Can you work these out from the model? Positions are in its coordinate system, mm. Face numbers are marked on the shaded views. A direction names the side the tool comes from. Give positions to 0.01 mm unless a question says otherwise; leave off trailing zeros. Loops run counter-clockwise (first coordinate to the right, second up) from the corner with the lowest first, then second, coordinate; pieces in that order, holes last.
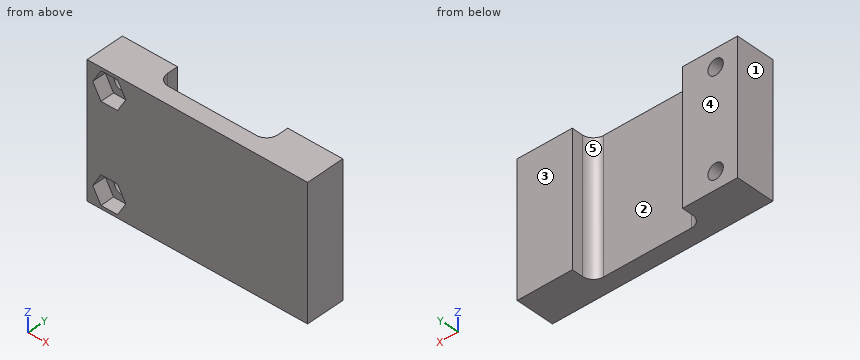
from build123d import *

# Parameters (mm, degrees)
SKETCH1_W           = 40
SKETCH1_H           = 24
SKETCH1_R           = 1.4
BOSS_EXTRUDE1_DEPTH = 7
SKETCH2_W           = 20
SKETCH2_H           = 24
CUT_EXTRUDE1_DEPTH  = 4
FILLET1_R           = 2
CUT_EXTRUDE2_DEPTH  = 2.5


with BuildPart() as part:
    # Sketch1 → Boss-Extrude1 (new body)
    with BuildSketch(Plane(origin=(0, 0, 0), x_dir=(1, 0, 0), z_dir=(0, 1, 0))):
        Rectangle(SKETCH1_W, SKETCH1_H)
        with Locations(Location((-16, 8.825, 0), (0, 0, 270))):
            Circle(SKETCH1_R, mode=Mode.SUBTRACT)
        with Locations(Location((-16, -8.825, 0), (0, 0, 270))):
            Circle(SKETCH1_R, mode=Mode.SUBTRACT)
    extrude(amount=BOSS_EXTRUDE1_DEPTH)

    # Sketch2 → Cut-Extrude1 (cut)
    with BuildSketch(Plane(origin=(0, 7, 0), x_dir=(1, 0, 0), z_dir=(0, 1, 0))):
        Rectangle(SKETCH2_W, SKETCH2_H)
    extrude(amount=-CUT_EXTRUDE1_DEPTH, mode=Mode.SUBTRACT)

    # Fillet1
    fillet1_edges = [part.edges().sort_by_distance(p)[0] for p in [
        (-10, 3, 0),
        (10, 3, 0),
    ]]
    fillet(fillet1_edges, radius=FILLET1_R)

    # Sketch3 → Cut-Extrude2 (cut)
    with BuildSketch(Plane.XZ):
        Polygon((-14.4988893, 6.225), (-12.9977786, 8.825), (-14.4988893, 11.425), (-17.5011107, 11.425), (-19.0022214, 8.825), (-17.5011107, 6.225), align=None)
        Polygon((-14.4988893, -11.425), (-12.9977786, -8.825), (-14.4988893, -6.225), (-17.5011107, -6.225), (-19.0022214, -8.825), (-17.5011107, -11.425), align=None)
    extrude(amount=-CUT_EXTRUDE2_DEPTH, mode=Mode.SUBTRACT)


solid = part.part
(1) Suppose I cut it at D-D on z = 9.75. List the corners of the cut face in (x, y) for me, plus the area to 3 significant figures.
Returned:
outline: (-20, 0) - (-18.47, 0) - (-18.47, 2.5) - (-17.05, 2.5) - (-17.05, 7) - (-20, 7) - close; (-14.95, 2.5) - (-13.53, 2.5) - (-13.53, 0) - (20, 0) - (20, 7) - (10, 7) - (10, 5) arc R2 cw to (8, 3) - (-8, 3) arc R2 cw to (-10, 5) - (-10, 7) - (-14.95, 7) - close
area: 180 mm2
(2) Will these pins go through, and if not, where does the flat tip stop? P1, Ø5, axis at x = 2.5, z = 5.5, coming from the +Y side; P2, Ø1.5, axis at x = 8.5, z = 7, coming from the -Y side; P3, Ø4.5, axis at x = -16, z = -8.825, coming from the -Y side; P4, Ø2.5, axis at x = -16, z = 8.825, coming from the +Y side.
Returned:
P1: stops at y = 3
P2: stops at y = 0
P3: stops at y = 2.5
P4: passes through
(3) Thinking about a two-plate mould opening in X: for the marked faces 1, 2 and 3, which applies, pulls with the +X half, pulls with the -X half, needs draft (parallel to the pull), parting line crosses it, or undercut?
Returned:
face 1: pulls with the -X half
face 2: undercut
face 3: needs draft
(4) Suppose I cut it at A-A on y = 6.25. List the corners of the cut face in (x, z) for me (3 decimals).
Returned:
outline: (-20, -12) - (-10, -12) - (-10, 12) - (-20, 12) - close; (10, -12) - (20, -12) - (20, 12) - (10, 12) - close; hole circle Ø2.8 at (-16, -8.825); hole circle Ø2.8 at (-16, 8.825)
(5) Suppose I cut it at B-B on x = -16. List the corners of the cut face in (y, z) for me (3 decimals).
Returned:
outline: (0, -12) - (7, -12) - (7, -10.225) - (2.5, -10.225) - (2.5, -11.425) - (0, -11.425) - close; (0, -6.225) - (2.5, -6.225) - (2.5, -7.425) - (7, -7.425) - (7, 7.425) - (2.5, 7.425) - (2.5, 6.225) - (0, 6.225) - close; (0, 11.425) - (2.5, 11.425) - (2.5, 10.225) - (7, 10.225) - (7, 12) - (0, 12) - close
(6) Suppose I cut it at C-C on y = 1.25. List the corners of the cut face in (x, z) for me (3 decimals), plus the area to 3 significant figures.
Returned:
outline: (-20, -12) - (20, -12) - (20, 12) - (-20, 12) - close; hole (-19.002, -8.825) - (-17.501, -11.425) - (-14.499, -11.425) - (-12.998, -8.825) - (-14.499, -6.225) - (-17.501, -6.225) - close; hole (-19.002, 8.825) - (-17.501, 6.225) - (-14.499, 6.225) - (-12.998, 8.825) - (-14.499, 11.425) - (-17.501, 11.425) - close
area: 913 mm2
(7) Which directions (+Z, -Z, +X, -X, +Y, -Y) give clear straight access to the entire face, cutting with the end or side of a thin tool? Please do the marked faces 4 and 5.
Returned:
face 4: +Z, -Z, +X, -X, +Y
face 5: +Z, -Z, +Y
(8) Please list where these lines run through material, in increasing order: probe 1 along Z at (x, y) = (-16, 5.2) (3 decimals); probe 2 along X at (y, z) = (6.75, -4.5); probe 3 along Y at (x, z) = (1.5, -4.75).
Returned:
probe 1: z = -12 to -10.225, -7.425 to 7.425, 10.225 to 12
probe 2: x = -20 to -10, 10 to 20
probe 3: y = 0 to 3
